Geometry: see drawing. Coordinates: mm, zero at the bounding-box minimum. A direction names the side the tool comes from. Give positions to 0.01 mm unless a question says otherwise; leave off trailing zeros. Order: outer loops, then holes, each group sorted by start corner. A loop starts at its lowest first (then second) coordinate and runs counter-clockwise, first axis right, second up. Notation, with made-up numbers: M -25,-6.5 L -19,-6.5 A13 cw -19,-2.5 Z; hole C 40,-40 d7. An arc over 180 degrees is marked long. Return JSON: item names as keys, results as strings.
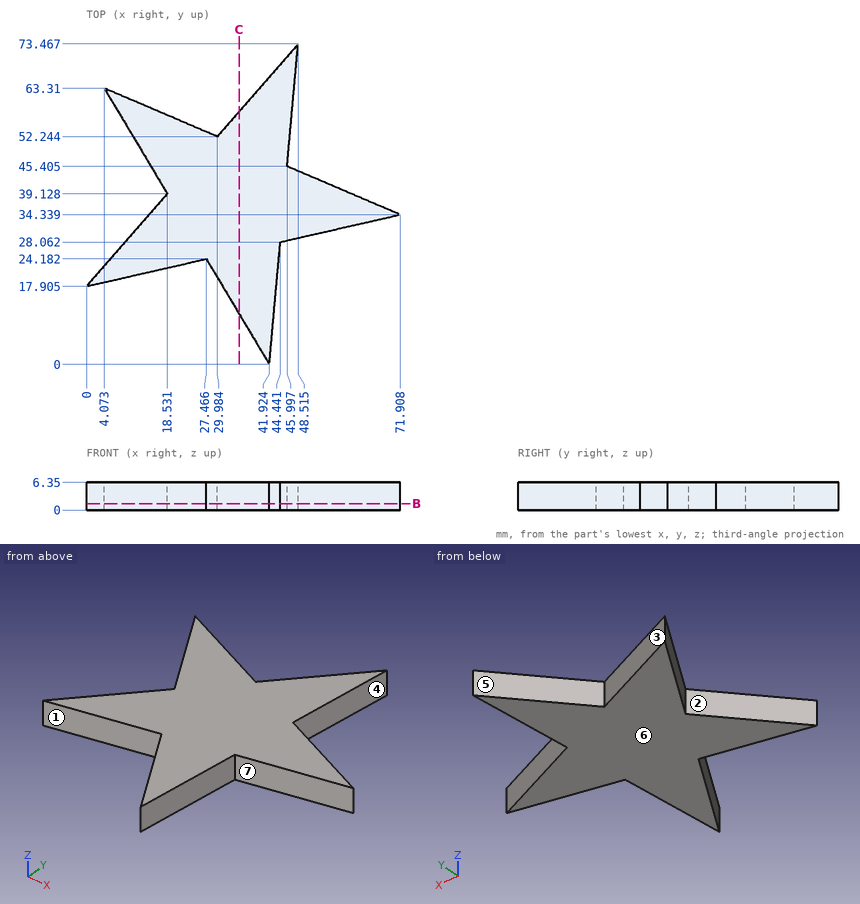
1. Section query C-C (x = 35). Return loops of the section in (y, z), then the cut area to 3 significant figures.
Evaluation:
{"outline": "M 11.58,0 L 57.99,0 L 57.99,6.35 L 11.58,6.35 Z", "area": "295 mm^2"}
2. Ray query, probe 1 along Y at (x, z) = (11.5, 3.5) (1 decimal); probe 2 along Y at (x, z) = (9, 3.25) (1 decimal); probe 3 along X at (y, z) = (38.5, 6.25) (1 decimal). Return the intervals inside material, ascending.
Evaluation:
{"probe 1": "y = 20.5 to 31.1, 50.9 to 60.1", "probe 2": "y = 20 to 28.2, 55.1 to 61.2", "probe 3": "x = 18 to 62.2"}
3. Draft query along Y for the marked faces 4, 5, 6 and 7. Return one class per face: pulls with the +Y half, pulls with the -Y half, needs draft (parallel to the pull), parting line crosses it, or undercut.
Evaluation:
{"face 4": "undercut", "face 5": "pulls with the +Y half", "face 6": "needs draft", "face 7": "pulls with the -Y half"}
4. Set-up query: the marked faces 1, 2 and 3. Return all of +Z, -Z, +X, -X, +Y, -Y with unobstructed straight access to the full face (end or side cutting, diameter ignored); none if empty.
Evaluation:
{"face 1": "+Z, -Z, -Y", "face 2": "+Z, -Z, -X", "face 3": "+Z, -Z, +Y"}
5. First-contact query: pin 1 (3 mm diameter, centred on y = 64.5, z = 1.5, fed in from -X); pin 2 (1.5 mm diameter, centred on y = 48, z = 5, fed in from -X); pin 3 (1 mm diameter, centred on x = 9.5, y = 30, fed in from +Z); pin 4 (3 mm diameter, centred on y = 50.5, z = 3, fed in from +X). Flat tips, straight axial feed; report the tip coordinate or a pass-through.
Evaluation:
{"pin 1": "stops at x = 4.07", "pin 2": "stops at x = 12.78", "pin 3": "passes through", "pin 4": "stops at x = 46.59"}
6. Section query B-B (z = 1.5). Return loops of the section in (x, y) (1 decimal).
Evaluation:
{"outline": "M 0,17.9 L 27.5,24.2 L 41.9,0 L 44.4,28.1 L 71.9,34.3 L 46,45.4 L 48.5,73.5 L 30,52.2 L 4.1,63.3 L 18.5,39.1 Z"}
